Autodesk Inventor part; units mm, degrees
ref_plane "YZ-Ebene" through (0, 0, 0) normal (1, 0, 0) x (0, 1, 0)
ref_plane "XZ-Ebene" through (0, 0, 0) normal (0, 1, 0) x (-1, 0, 0)
ref_plane "XY-Ebene" through (0, 0, 0) normal (0, 0, 1) x (1, 0, 0)
sketch "Skizze1" plane through (0, 0, 0) normal (0, 0, 1) x (1, 0, 0)
  line L0 (-3.78, 0) -> (3.78, 0)
  line L1 (0, -4.3648) -> (0, 4.3648)
  line L2 (0, 3.1177) -> (2.7, 1.5588)
  line L3 (2.7, 1.5588) -> (2.7, -1.5588)
  line L4 (2.7, -1.5588) -> (0, -3.1177)
  line L5 (0, -3.1177) -> (-2.7, -1.5588)
  line L6 (-2.7, -1.5588) -> (-2.7, 1.5588)
  line L7 (-2.7, 1.5588) -> (0, 3.1177)
  point P0 (0, 0)
  point P1 (0, 0)
  dimension "d0" = 5.4
extrude "Extrusion1" add sketch "Skizze1" along normal blind 1.6
sketch "Skizze2" plane through (0, 0, 1.6) normal (0, 0, 1) x (1, 0, 0)
  line L0 (0, 3.1177) -> (-2.7, 1.5588)
  circle A0 centre (0, 0) radius 2.7
extrude "Extrusion2" cut sketch "Skizze2" against normal blind 1.5 draft 45 keep common part
sketch "Skizze3" plane through (0, 0, 1.6) normal (0, 0, 1) x (1, 0, 0)
  arc A0 (-2.7, 0) -> (-1.35, -2.3383) centre (0, 0) ccw
  circle A1 centre (0, 0) radius 1.25
  dimension "d5" = 2.5
extrude "Extrusion3" cut sketch "Skizze3" against normal blind 1.5
thread "Gewinde1"
properties part number "Mutter_ra8846s" material "Stahl"
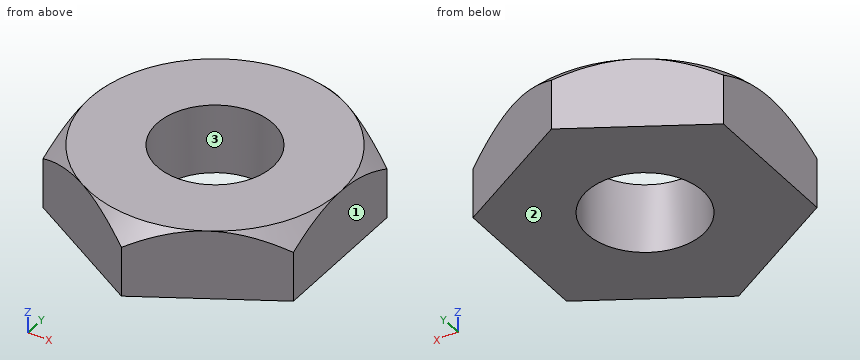
Verification items for the finished model (mm, model axes). Face numbers are marked on the shaded views. Give positions to 0.01 mm unless a question says otherwise; leave off trailing zeros. Order: outer loops, then holes, each group sorted by start corner. A loop starts at its lowest first (then second) coordinate and runs counter-clockwise, first axis right, second up. Notation, with made-up numbers: M -40,-28 L 16,-28 A19 cw 16,-14 Z; hole C -28.75,-4 d7. An arc over 180 degrees is marked long. Answer as a JSON object with one key per item and string values. Group by question number.
1) Cross-section at B-B (z = 1.35). Enter the section's corners in (x, y), then the cut area to 3 significant figures.
2) Mould release check, pull along X, two halves, no side actions. Record for the marked faces 1, 2 and 3: released by +X, released by -X, zero draft, split by the parting line, or undercut.
3) Cross-section at A-A (z = 0.6). Enter the section's corners in (x, y).
4) Scan lines: line 1 along X through (y, z) = (-0.5, 0.4); line 2 along X through (y, z) = (-0.75, 0.5); line 3 along Y through (x, z) = (-0.95, 0.7). Record each from-to range of solid material in increasing order. Write a range as [from, to].
Result sheet:
{
 "1": {"outline": "M -2.7,-1.19 A2.95 ccw -2.38,-1.74 L -0.32,-2.93 A2.95 ccw 0.32,-2.93 L 2.38,-1.74 A2.95 ccw 2.7,-1.19 L 2.7,1.19 A2.95 ccw 2.38,1.74 L 0.32,2.93 A2.95 ccw -0.32,2.93 L -2.38,1.74 A2.95 ccw -2.7,1.19 Z; hole C 0,0 d2.5", "area": "20.0 mm2"},
 "2": {"face 1": "released by +X", "face 2": "zero draft", "face 3": "undercut"},
 "3": {"outline": "M -2.7,-1.56 L 0,-3.12 L 2.7,-1.56 L 2.7,1.56 L 0,3.12 L -2.7,1.56 Z; hole C 0,0 d2.5"},
 "4": {"line 1": "x = [-2.7, -1.15], [1.15, 2.7]", "line 2": "x = [-2.7, -1], [1, 2.7]", "line 3": "y = [-2.57, -0.81], [0.81, 2.57]"}
}
